Solid Edge part; units mm, degrees
sketch "Sketch1" plane through (0, 0, 4) normal (0, 0, 1) x (1, 0, 0)
  line L0 (0, 17.5) -> (0, -17.5)
  line L1 (0, -17.5) -> (35, -17.5)
  line L2 (35, -17.5) -> (70.5843, -10.4379)
  line L3 (70.5843, 10.4379) -> (70.5843, -10.4379)
  line L4 (35, 17.5) -> (70.5843, 10.4379)
  line L5 (35, 17.5) -> (0, 17.5)
  dimension "D1" = 35
extrude "ExtrudedProtrusion_1" add sketch "Sketch1" along normal blind 2
sketch "Sketch2" plane through (38.9148, 0, 6) normal (0, 0, 1) x (0, 1, 0)
  circle A0 centre (0, 24.5181) radius 5
extrude "Cutout1" cut sketch "Sketch2" against normal through all
sketch "Sketch3" plane through (35.2922, 0, 4) normal (0, 0, -1) x (0, -1, 0)
  circle A0 centre (10, 26.4824) radius 1
  circle A1 centre (-5, -30.9693) radius 1
  circle A2 centre (5, -30.9693) radius 1
  circle A3 centre (-10, 26.4824) radius 1
  dimension "D1" = 5
extrude "Cutout2" cut sketch "Sketch3" against normal through all
properties material "Polypropylene, high impact"
Design review of the part built by this model. Coordinates are the model's own, in mm. Give positions to 0.01 mm unless a question says otherwise; leave off trailing zeros. Order: outer loops, then holes, each group sorted by start corner. A loop starts at its lowest first (then second) coordinate and runs counter-clockwise, first axis right, second up. Notation, with made-up numbers: (-17.5, -15.5) - (10.5, -15.5) arc R24 ccw to (10.5, 12.5) - close; hole circle Ø6 at (78, 19). An arc over 180 degrees is marked (long way). Write item = value, one per line. Start each with the question number.
Q1. We need section A-A on y = 0. State the section outline as (x, z) points, plus the area to 3 significant figures.
Q2. To check wall thickness, follow L1, parallel to X at y = 0, z = 5.35; L2, parallel to X at y = -10, z = 5; L3, parallel to Y at x = 11, z = 5.4. State the ranges of each line that lie inside material, in increasing order. Write a range as from..to.
Q3. We need section D-D on x = 47. State the section outline as (y, z) points.
Q4. Clearance check with a flat-ended pin moving along its axis: pin 1 Ø1.2 at (x, y) = (8.81, -10) entering from +Z. State where the tip first meets the part, or that it passes through.
Q5. We need section B-B on z = 4.6. State the section outline as (x, y) points.
Q6. Mouldability with a two-part tool opening along Y and no side actions: class faces 1 (the face through (19.28, -1.08, 5.01)), 2 (the face through (70.584, 0, 5)), 3 (the face through (18, 17.5, 5)) as released by +Y, released by -Y, zero draft, split by the parting line, or undercut.
Q7. We need section C-C on y = -12. State the section outline as (x, z) points.
Working result:
q1.outline = (0, 4) - (9.4, 4) - (9.4, 6) - (0, 6) - close; (19.4, 4) - (70.58, 4) - (70.58, 6) - (19.4, 6) - close
q1.area = 121 mm²
q2.L1 = 0..9.4, 19.4..70.58
q2.L2 = 0..7.81, 9.81..70.58
q2.L3 = -17.5..-3.67, 3.67..17.5
q3.outline = (-15.12, 4) - (15.12, 4) - (15.12, 6) - (-15.12, 6) - close
q4.pin_1 = through
q5.outline = (0, -17.5) - (35, -17.5) - (70.58, -10.44) - (70.58, 10.44) - (35, 17.5) - (0, 17.5) - close; hole circle Ø2 at (8.81, -10); hole circle Ø2 at (8.81, 10); hole circle Ø10 at (14.4, 0); hole circle Ø2 at (66.26, -5); hole circle Ø2 at (66.26, 5)
q6.face_1 = undercut
q6.face_2 = zero draft
q6.face_3 = released by +Y
q7.outline = (0, 4) - (62.71, 4) - (62.71, 6) - (0, 6) - close
